Verification items for this drawing (mm, ordinates from the low corner). A direction names the side the tool comes from. Give positions to 0.01 mm unless a question says otherwise; leave off trailing zeros. Loops run counter-clockwise (first coordinate to the right, second up) from the corner with the lowest first, then second, coordinate; pieces in that order, holes last. Notation, with made-up numbers: M -2.5,53.5 L 22.5,53.5 A25 cw 22.5,83.5 Z; hole C 60.5,-34 d5. An arc over 180 degrees is marked long. Use one line per item in the form item = value.
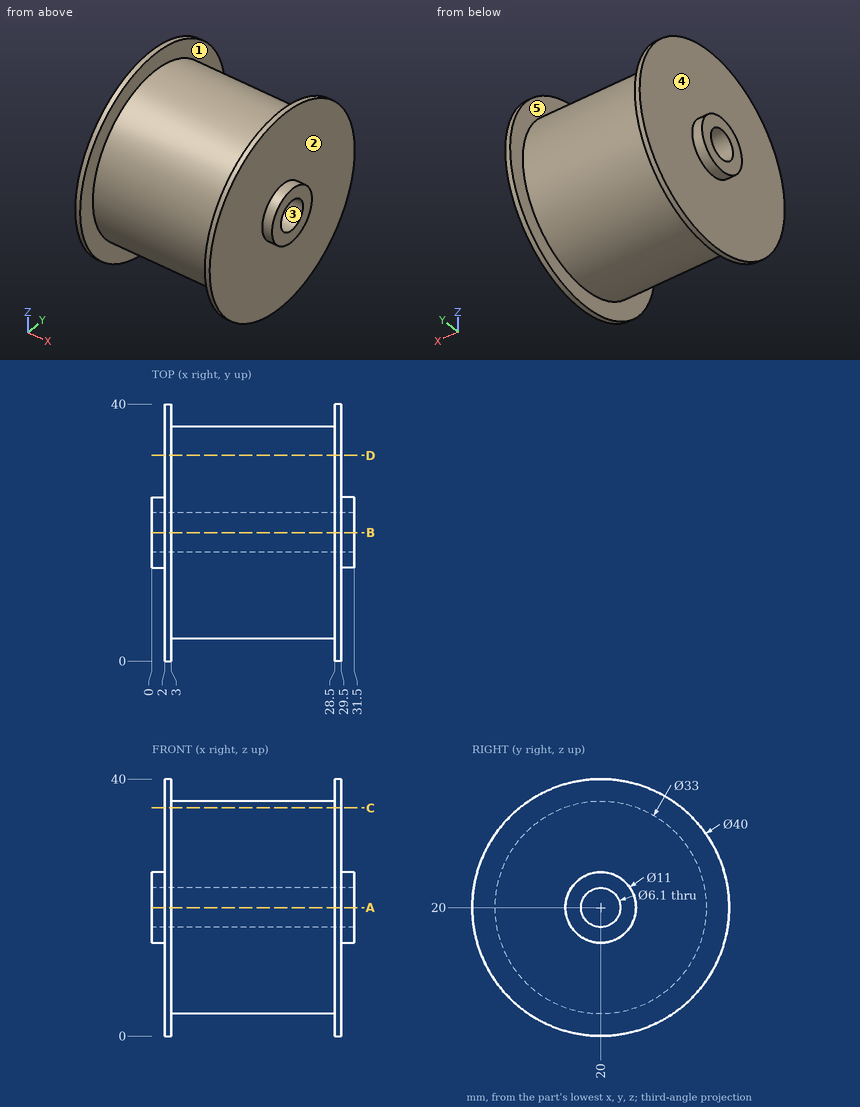
1) Section check D-D (y = 32). Record the cut outline in (x, z), then the cut area to 3 significant figures.
Evaluation:
outline = M 2,4 L 3,4 L 3,8.68 L 28.5,8.68 L 28.5,4 L 29.5,4 L 29.5,36 L 28.5,36 L 28.5,31.32 L 3,31.32 L 3,36 L 2,36 Z
area = 642 mm^2
2) Release check for a two-part mould opening along X. For the marked faces 3, 4 and 5 record: pulls with the +X half, pulls with the -X half, needs draft (parallel to the pull), parting line crosses it, or undercut.
Evaluation:
face_3 = needs draft
face_4 = pulls with the -X half
face_5 = undercut
3) Section check A-A (z = 20). Record the cut outline in (x, y).
Evaluation:
outline = M 0,14.5 L 2,14.5 L 2,0 L 3,0 L 3,3.5 L 28.5,3.5 L 28.5,0 L 29.5,0 L 29.5,14.5 L 31.5,14.5 L 31.5,16.95 L 0,16.95 Z; M 0,23.05 L 31.5,23.05 L 31.5,25.5 L 29.5,25.5 L 29.5,40 L 28.5,40 L 28.5,36.5 L 3,36.5 L 3,40 L 2,40 L 2,25.5 L 0,25.5 Z
4) Scan lines: line 1 (Z direction, x = 16, y = 20); line 2 (X direction, y = 5, z = 13); line 3 (X direction, y = 32.5, z = 10.5). Record each from-to range of solid material in increasing order.
Evaluation:
line_1 = 3.5 to 16.95, 23.05 to 36.5
line_2 = 2 to 3, 28.5 to 29.5
line_3 = 2 to 29.5
5) Section check C-C (z = 35.5). Record the cut outline in (x, y), then the cut area to 3 significant figures.
Evaluation:
outline = M 2,7.36 L 3,7.36 L 3,14.34 L 28.5,14.34 L 28.5,7.36 L 29.5,7.36 L 29.5,32.64 L 28.5,32.64 L 28.5,25.66 L 3,25.66 L 3,32.64 L 2,32.64 Z
area = 339 mm^2
6) Depth check by flat-ended pin: pin 1 Ø2 at (x, y) = (22, 4.5) entering from -Z; pin 2 Ø1 at (x, y) = (24, 8.5) entering from +Z; pin 3 Ø3 at (y, z) = (32, 9) entering from -X. Enter the tip coordinate at first touch or a pass-through.
Evaluation:
pin_1 = 12.13
pin_2 = 32.3
pin_3 = 2
7) Set-up check for the marked faces 1 and 2: record each of +Z, -Z, +X, -X, +Y, -Y from which the full face is reachable in a straight line by a thin tool's end or side.
Evaluation:
face_1 = none
face_2 = +X
